Can you work these out from the model? Positions are in its coordinate system, mm. Coordinates: 2 decimals unless noted, no trailing zeros. Order: outer loops, then holes, each group sorted by start corner. A loop starts at its lowest first (then second) coordinate and runs counter-clockwise, first axis right, second up. Notation, with made-up numbers: (24.5, 31.25) -> (67.5, 31.25) arc R14 ccw to (67.5, 41.25) -> close; hole circle Ø8 at (-7, -37). An arc over 180 degrees is marked (long way). Answer in a Markdown table with one row per item. Add a question column.
1. Imagine slicing it at D-D on x = 92. Write out the boundary of the cut face in (y, z), plus the area to 3 significant figures.
2. If I drill on line 1 along Y through (x, z) = (-41, 26); line 2 along Y through (x, z) = (-132, 34), over which ranges is the centre line in solid material (lowest first)? Write a range as [from, to].
3. Will this pin go through, and if not, where does the flat tip stop? pin 1 (5 mm diameter, centred on x = -79.64, y = 116.83, fed in from -Z).
4. Imagine slicing it at A-A on x = -58. Write out the boundary of the cut face in (y, z), plus the area to 3 significant figures.
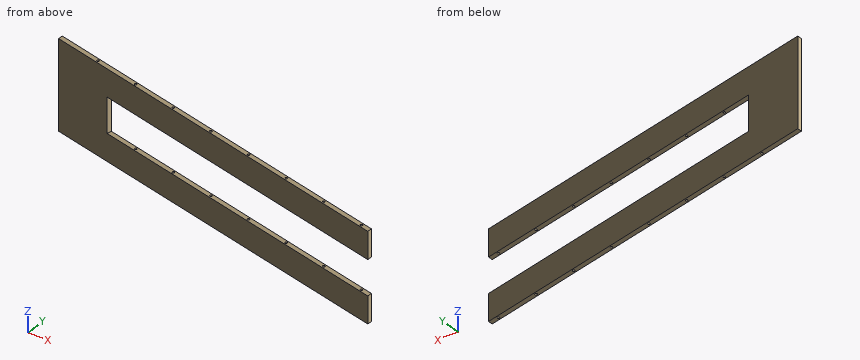
Autodesk Inventor part; units mm, degrees
ref_plane "Work Plane3" through (111499.6524, -24907.1137, 0) normal (-0.2188346, -0.975762, 0) x (0, 0, -1)
ref_plane "YZ Plane" through (0, 0, 0) normal (1, 0, 0) x (0, 1, 0)
ref_plane "XZ Plane" through (0, 0, 0) normal (0, 1, 0) x (-1, 0, 0)
sketch "Sketch4" plane through (0, 0, 0) normal (0, 0, 1) x (1, 0, 0)
  line L0 (293.2796, 30.0061) -> (-199.5823, 140.5264)
  line L1 (293.2796, 36.3718) -> (-199.5823, 146.9202)
  line L2 (-199.5823, 146.9202) -> (-199.5823, 140.5264)
  line L3 (293.2796, 30.0061) -> (-199.5823, 140.5264)
  line L4 (293.2796, 36.3718) -> (-199.5823, 146.9202)
  line L5 (-199.5823, 146.9202) -> (-199.5823, 140.5264)
  line L6 (293.2796, 30.0061) -> (293.2796, 36.3718)
sketch "Sketch5" plane through (0, 0, 0) normal (0, 0, 1) x (1, 0, 0)
  circle A0 centre (280.3828, 36.0784) radius 3.5
  circle A1 centre (220.3828, 49.5364) radius 3.5
  circle A2 centre (160.3828, 62.9943) radius 3.5
  circle A3 centre (100.3828, 76.4523) radius 3.5
  circle A4 centre (40.3604, 89.9135) radius 3.5
  circle A5 centre (-139.6396, 130.2873) radius 3.5
  circle A6 centre (-79.6396, 116.8294) radius 3.5
  circle A7 centre (-19.6396, 103.3714) radius 3.5
extrude "Extrusion3" add sketch "Sketch4" along normal blind 115.75
ref_plane "Work Plane3" through (111499.6524, -24907.1137, 0) normal (-0.2188346, -0.975762, 0) x (0, 0, -1)
sketch "Sketch6" plane through (111499.6524, -24907.1137, 0) normal (-0.2188346, -0.975762, 0) x (0, 0, -1)
  line L0 (0, -114474.0796) -> (-115.4577, -114474.0796)
  line L1 (-115.4577, -114474.0796) -> (-115.4577, -113968.0685)
  line L2 (-115.4577, -113968.0685) -> (0, -113968.0685)
  line L3 (0, -113968.0685) -> (0, -114474.0796)
  line L4 (0, -113968.0539) -> (-115.75, -113968.0539)
  line L5 (-27.7607, -113968.0539) -> (-91.2309, -113968.0539)
  line L6 (-75.4577, -113983.6101) -> (-36.9803, -113983.6101)
  line L7 (-35, -113968.0685) -> (-80.4577, -113968.0685)
  line L8 (-80.4577, -113968.0685) -> (-80.4577, -114394.0796)
  line L9 (-80.4577, -114394.0796) -> (-35, -114394.0796)
  line L10 (-35, -114394.0796) -> (-35, -113968.0685)
  point P0 (0, -114247.6585)
  dimension "d28" = 506.0111
  dimension "d29" = 115.4577
  dimension "d30" = 35
  dimension "d32" = 80
  dimension "d42" = 35
emboss "Emboss1" sketch "Sketch6" operation cut depth 8 direction (-0.2188346, -0.975762, 0) contours L10 L9 L8 L2
hole "Hole1" at (-139.6396, 130.2873, 0) at (-79.6396, 116.8294, 0) at (-19.6396, 103.3714, 0) at (40.3604, 89.9135, 0) at (100.3828, 76.4523, 0) at (160.3828, 62.9943, 0) at (220.3828, 49.5364, 0) at (280.3828, 36.0784, 0) direction (0, 0, 1) diameter 3 end through all
equation "\"d40\" = Thickness"
equation "\"BendRadius\" = Thickness"
equation "\"BendReliefWidth\" = Thickness"
equation "\"BendReliefDepth\" = 0.5 * Thickness"
equation "\"CornerReliefSize\" = 4 * Thickness"
equation "\"MinimumRemnant\" = 2 * Thickness"
equation "\"TransitionRadius\" = BendRadius"
equation "\"JacobiRadiusSize\" = BendRadius"
equation "\"GapSize\" = Thickness"
properties part number "sidesupport"
Answers follow:
| question | item | result |
|---|---|---|
| 1 | outline | (75.14, 0) -> (81.52, 0) -> (81.52, 35) -> (75.14, 35) -> close; (75.14, 80.46) -> (81.52, 80.46) -> (81.52, 115.75) -> (75.14, 115.75) -> close |
| 1 | area | 448 mm² |
| 2 | line 1 | y = [104.97, 111.35] |
| 2 | line 2 | y = [125.37, 131.76] |
| 3 | pin 1 | stops at z = 0 |
| 4 | outline | (108.78, 0) -> (115.16, 0) -> (115.16, 35) -> (108.78, 35) -> close; (108.78, 80.46) -> (115.16, 80.46) -> (115.16, 115.75) -> (108.78, 115.75) -> close |
| 4 | area | 449 mm² |
